from build123d import *

# Parameters (mm, degrees)
BOSS_EXTRUDE1_DEPTH     = 1026
CUT_EXTRUDE1_DEPTH      = 30126.076908122
CUT_EXTRUDE1_DEPTH_BACK = 30126.076908122
SKETCH2_R               = 11


with BuildPart() as part:
    # Sketch1 → Boss-Extrude1 (new body)
    with BuildSketch(Plane(origin=(0, 0, 0), x_dir=(0, 0, -1), z_dir=(1, 0, 0))):
        Polygon((-29120.788440545, 7606.867460507), (-29091.195271738, 7606.867460507), (-28962.788440545, 7645.080988537), (-28795.480129553, 7606.801691282), (-28796.288440545, 7601.867460507), (-28962.788440545, 7640.014342662), (-29090.788440545, 7601.867460507), (-29120.788440545, 7601.867460507), align=None)
    extrude(amount=BOSS_EXTRUDE1_DEPTH)

    # Sketch2 → Cut-Extrude1 (cut, two sides: drawn at the far end of the back side and taken through both)
    with BuildSketch(Plane(origin=(0, 0, 0), x_dir=(1, 0, 0), z_dir=(0, 1, 0)).offset(-CUT_EXTRUDE1_DEPTH_BACK)):
        with Locations(Location((50, -28962.788440545, 0), (0, 0, 180))):
            Circle(SKETCH2_R)
        with Locations(Location((150, -28962.788440545, 0), (0, 0, 180))):
            Circle(SKETCH2_R)
        with Locations(Location((392, -28962.788440545, 0), (0, 0, 180))):
            Circle(SKETCH2_R)
        with Locations(Location((634, -28962.788440545, 0), (0, 0, 180))):
            Circle(SKETCH2_R)
        with Locations(Location((876, -28962.788440545, 0), (0, 0, 180))):
            Circle(SKETCH2_R)
        with Locations(Location((976, -28962.788440545, 0), (0, 0, 180))):
            Circle(SKETCH2_R)
    extrude(amount=CUT_EXTRUDE1_DEPTH + CUT_EXTRUDE1_DEPTH_BACK, mode=Mode.SUBTRACT)


solid = part.part
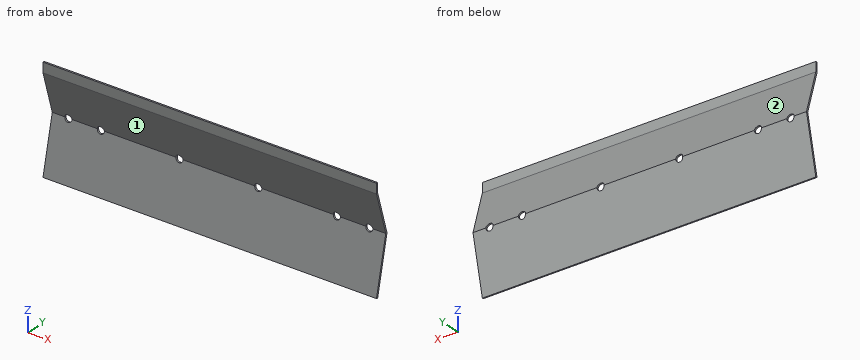
Geometry check sheet. Reference: the model listing, model coordinates, mm. Face numbers are marked on the shaded views. A direction names the side the tool comes from. Give positions to 0.01 mm unless a question says otherwise; leave off trailing zeros. Loops run counter-clockwise (first coordinate to the right, second up) from the corner with the lowest first, then second, coordinate; pieces in that order, holes last. Notation, with made-up numbers: M 1.5,-17.75 L 42.5,-17.75 A11 ccw 42.5,-12.75 Z; hole C -5.5,61 d4. An arc over 180 degrees is marked long. Answer as a JSON object with one key per item and string values. Group by question number.
Item 1: Sectioned sample at C-C on x = 976. Record the boundary of the cut face in (y, z).
Item 2: Access from +Z, -Z, +X, -X, +Y, -Y to the whole of each face (thin tool, end or side, straight path). Record for the marked faces 1 and 2.
Item 3: Material ranges on L1, parallel to Y at x = 169, z = 29101; L2, parallel to Y at x = 680.5, z = 28818, recorded low to high.
Item 4: Sectioned sample at A-A on x = 827. Record the boundary of the cut face in (y, z), plus the area to 3 significant figures.
Item 5: Gauge pin test, flat ends, axial feed: pin 1 (8 mm diameter, centred on x = 847, z = 28900.5, fed in from +Y); pin 2 (12 mm diameter, centred on x = 625.5, z = 29067, fed in from -Y); pin 3 (4 mm diameter, centred on x = 257, z = 28886.5, fed in from -Y). Record the tip position at first contact, or that the pin passes through.
Item 6: Sectioned sample at B-B on y = 7623. Record the boundary of the cut face in (x, z), plus the area to 3 significant figures.
Item 7: Sectioned sample at D-D on z = 29024.5. Record the boundary of the cut face in (x, y).
Findings below:
{
 "1": {"outline": "M 7601.87,28796.29 L 7606.8,28795.48 L 7642.56,28951.79 L 7637.49,28951.79 Z; M 7601.87,29090.79 L 7636.74,28973.79 L 7641.81,28973.79 L 7606.87,29091.2 L 7606.87,29120.79 L 7601.87,29120.79 Z"},
 "2": {"face 1": "+X, -X, -Y", "face 2": "+Z, +X, -X, +Y"},
 "3": {"L1": "7601.87 to 7606.87", "L2": "7606.84 to 7611.95"},
 "4": {"outline": "M 7601.87,28796.29 L 7606.8,28795.48 L 7645.08,28962.79 L 7606.87,29091.2 L 7606.87,29120.79 L 7601.87,29120.79 L 7601.87,29090.79 L 7640.01,28962.79 Z", "area": "1,650 mm2"},
 "5": {"pin 1": "y = 7631.74", "pin 2": "y = 7607.17", "pin 3": "y = 7622.08"},
 "6": {"outline": "M 0,28866.28 L 1026,28866.28 L 1026,28888.53 L 0,28888.53 Z; M 0,29019.88 L 1026,29019.88 L 1026,29036.99 L 0,29036.99 Z", "area": "40,400 mm2"},
 "7": {"outline": "M 0,7621.62 L 1026,7621.62 L 1026,7626.72 L 0,7626.72 Z"}
}
